from build123d import *

# Parameters (mm, degrees)
SKETCH1_W           = 52
SKETCH1_H           = 11
BOSS_EXTRUDE1_DEPTH = 12
SKETCH3_W           = 12
SKETCH3_H           = 8
CUT_REVOLVE1_ANGLE  = 90
SKETCH4_W           = 13
SKETCH4_H           = 4
BOSS_EXTRUDE2_DEPTH = 17.603
CUT_EXTRUDE1_DEPTH  = 60.884318557
SKETCH7_R           = 1.5
CUT_EXTRUDE2_DEPTH  = 60.884318557
SKETCH8_R           = 4.2
CUT_EXTRUDE3_DEPTH  = 3.5
SKETCH9_R           = 3
CUT_EXTRUDE4_DEPTH  = 7.5
SKETCH10_R          = 1.6
CUT_EXTRUDE5_DEPTH  = 61.358359893
SKETCH11_R          = 1.5
CUT_EXTRUDE6_DEPTH  = 61.548588827
SKETCH13_R          = 3
CUT_EXTRUDE7_DEPTH  = 10
CHAMFER3_SIZE       = 0.5
FILLET11_R          = 3
FILLET12_R          = 3


with BuildPart() as part:
    # Sketch1 → Boss-Extrude1 (new body)
    with BuildSketch(Plane.XY):
        with Locations((26, 5.5)):
            Rectangle(SKETCH1_W, SKETCH1_H)
    extrude(amount=BOSS_EXTRUDE1_DEPTH)

    # Sketch3 → Cut-Revolve1 (revolve, cut)
    with BuildSketch(Plane.ZY):
        with Locations((6, 4)):
            Rectangle(SKETCH3_W, SKETCH3_H)
    revolve(axis=Axis((0, 0, 0), (0, 0, -1)), revolution_arc=CUT_REVOLVE1_ANGLE, mode=Mode.SUBTRACT)

    # Sketch4 → Boss-Extrude2 (add)
    with BuildSketch(Plane(origin=(0, 11, 0), x_dir=(1, 0, 0), z_dir=(0, 1, 0))):
        with Locations((45.5, -2)):
            Rectangle(SKETCH4_W, SKETCH4_H)
    extrude(amount=BOSS_EXTRUDE2_DEPTH)

    # Sketch6 → Cut-Extrude1 (cut, through all)
    with BuildSketch(Plane.XY.offset(4)):
        with BuildLine():
            ThreePointArc((45.5, 28.603), (50.096194078, 26.699194078), (52, 22.103))
            Line((52, 22.103), (52, 28.603))
            Line((52, 28.603), (45.5, 28.603))
        make_face()
        with BuildLine():
            Line((39, 28.603), (39, 22.103))
            ThreePointArc((39, 22.103), (40.903805922, 26.699194078), (45.5, 28.603))
            Line((45.5, 28.603), (39, 28.603))
        make_face()
    extrude(amount=-CUT_EXTRUDE1_DEPTH, mode=Mode.SUBTRACT)

    # Sketch7 → Cut-Extrude2 (cut, through all)
    with BuildSketch(Plane.XY.offset(4)):
        with Locations((47, 22.103)):
            Circle(SKETCH7_R)
    extrude(amount=-CUT_EXTRUDE2_DEPTH, mode=Mode.SUBTRACT)

    # Sketch8 → Cut-Extrude3 (cut)
    with BuildSketch(Plane.XY.offset(12)):
        with Locations((46.5, 5.5)):
            Circle(SKETCH8_R)
    extrude(amount=-CUT_EXTRUDE3_DEPTH, mode=Mode.SUBTRACT)

    # Sketch9 → Cut-Extrude4 (cut)
    with BuildSketch(Plane.XY.offset(8.5)):
        with Locations((46.5, 5.5)):
            Circle(SKETCH9_R)
    extrude(amount=-CUT_EXTRUDE4_DEPTH, mode=Mode.SUBTRACT)

    # Sketch10 → Cut-Extrude5 (cut, through all)
    with BuildSketch(Plane.XY.offset(1)):
        with Locations((46.5, 5.5)):
            Circle(SKETCH10_R)
    extrude(amount=-CUT_EXTRUDE5_DEPTH, mode=Mode.SUBTRACT)

    # Sketch11 → Cut-Extrude6 (cut, through all)
    with BuildSketch(Plane.XZ):
        with Locations(Location((37.5, 4.5, 0), (0, 0, 270))):
            Circle(SKETCH11_R)
        with Locations(Location((20.5, 4.5, 0), (0, 0, 270))):
            Circle(SKETCH11_R)
    extrude(amount=-CUT_EXTRUDE6_DEPTH, mode=Mode.SUBTRACT)

    # Sketch13 → Cut-Extrude7 (cut)
    with BuildSketch(Plane.XZ):
        with Locations(Location((37.5, 4.5, 0), (0, 0, 270))):
            Circle(SKETCH13_R)
    extrude(amount=-CUT_EXTRUDE7_DEPTH, mode=Mode.SUBTRACT)

    # Chamfer3
    chamfer3_edges = [part.edges().sort_by_distance(p)[0] for p in [
        (20.5, 11, 6),
        (20.5, 0, 6),
    ]]
    chamfer(chamfer3_edges, length=CHAMFER3_SIZE)

    # Fillet11
    fillet11_edges = [part.edges().sort_by_distance(p)[0] for p in [
        (0, 8, 6),
    ]]
    fillet(fillet11_edges, radius=FILLET11_R)

    # Fillet12
    fillet12_edges = [part.edges().sort_by_distance(p)[0] for p in [
        (8, 0, 6),
    ]]
    fillet(fillet12_edges, radius=FILLET12_R)


solid = part.part
Verification items for the finished model (mm, model axes). A direction names the side the tool comes from. Give positions to 0.01 mm unless a question says otherwise; leave off trailing zeros. Loops run counter-clockwise (first coordinate to the right, second up) from the corner with the lowest first, then second, coordinate; pieces in that order, holes last.
1. Cross-section at A-A on z = 4.5. Record the cut outline in (x, y).
Derived:
outline: (0, 10.58) arc R3 ccw to (2.18, 7.7) arc R8 cw to (7.7, 2.18) arc R3 ccw to (10.58, 0) - (18.5, 0) - (19, 0.5) - (19, 10.5) - (18.5, 11) - (0, 11) - close; (22, 0.5) - (22.5, 0) - (34.5, 0) - (34.5, 10) - (36, 10) - (36, 11) - (22.5, 11) - (22, 10.5) - close; (39, 10) - (40.5, 10) - (40.5, 0) - (52, 0) - (52, 11) - (39, 11) - close; hole circle Ø6 at (46.5, 5.5)
2. Go/stop test with flat-tipped pins: P1, Ø4, axis at x = 47, y = 22.103, coming from the +Z side; P2, Ø7, axis at x = 37.5, z = 4.5, coming from the +Y side; P3, Ø13.5, axis at x = 46.5, y = 5.5, coming from the +Z side; P4, Ø3, axis at x = 5.5, z = 9, coming from the +Y side. Record where each tip stops, or that it passes through.
Derived:
P1: stops at z = 4
P2: stops at y = 26.76
P3: stops at z = 12
P4: stops at y = 11
3. Tool access check on faces 5 (the cylindrical face through (45.5, 22.17, 2.03)), 6 (the cylindrical face through (43.5, 5.6, 4.8)), 7 (the flat face through (36, 10, 3)). Record the directions out of +Z, -Z, +X, -X, +Y, -Y that give a thin tool (end or side, any length) a straight path to the whole face; none if there is none.
Derived:
face 5: +Z, -Z
face 6: +Z
face 7: -Y
4. Cross-section at C-C on y = 5.5. Record the cut outline in (x, z).
Derived:
outline: (5.81, 0) - (44.9, 0) - (44.9, 1) - (43.5, 1) - (43.5, 8.5) - (42.3, 8.5) - (42.3, 12) - (5.81, 12) - close; (48.1, 0) - (52, 0) - (52, 12) - (50.7, 12) - (50.7, 8.5) - (49.5, 8.5) - (49.5, 1) - (48.1, 1) - close; hole circle Ø3 at (20.5, 4.5); hole circle Ø6 at (37.5, 4.5)
5. Release check for a two-part mould opening along X. For faces 1 (the flat face through (52, 8, 5)), 2 (the cylindrical face through (0.591, 8.796, 6.084)), 3 (the flat face through (45, 20, 4)), 4 (the flat face through (48, 4, 1)) record: +X half, -X half, draft (parallel to the pull), parting line (faces both ways), or undercut.
Derived:
face 1: +X half
face 2: -X half
face 3: draft
face 4: undercut
6. Material ranges on probe 1 along X at (y, z) = (10.45, 4.5); probe 2 along X at (y, z) = (6, 4.5); probe 3 along X at (y, z) = (8, 4.5), recorded low to high.
Derived:
probe 1: x = 0 to 19, 22 to 36, 39 to 52
probe 2: x = 5.29 to 19, 22 to 34.5, 40.5 to 43.54, 49.46 to 52
probe 3: x = 1.47 to 19, 22 to 34.5, 40.5 to 44.84, 48.16 to 52
7. Cross-section at D-D on z = 10. Record the cut outline in (x, y), and give its area (3 significant figures).
Derived:
outline: (0, 10.58) arc R3 ccw to (2.18, 7.7) arc R8 cw to (7.7, 2.18) arc R3 ccw to (10.58, 0) - (52, 0) - (52, 11) - (0, 11) - close; hole circle Ø8.4 at (46.5, 5.5)
area: 464 mm2
8. Cross-section at B-B on x = 37.5. Record the cut outline in (y, z), and give its area (3 significant figures).
Derived:
outline: (0, 0) - (11, 0) - (11, 3) - (10, 3) - (10, 1.5) - (0, 1.5) - close; (0, 7.5) - (10, 7.5) - (10, 6) - (11, 6) - (11, 12) - (0, 12) - close
area: 69.0 mm2
